from build123d import *

# Parameters (mm, degrees)
SKETCH1_R           = 3.25
BOSS_EXTRUDE1_DEPTH = 6
FILLET1_R           = 0.5
SCALE_1_SCALE       = 2


with BuildPart() as part:
    # Sketch1 → Boss-Extrude1 (new body)
    with BuildSketch(Plane.XY):
        with BuildLine():
            Line((-50.218340611, 5), (149.781659389, 5))
            ThreePointArc((149.781659389, 5), (154.781659389, 0), (149.781659389, -5))
            Line((149.781659389, -5), (-50.218340611, -5))
            ThreePointArc((-50.218340611, -5), (-55.218340611, 0), (-50.218340611, 5))
        make_face()
        with Locations((-50.218340611, 0)):
            Circle(SKETCH1_R, mode=Mode.SUBTRACT)
        with Locations((149.781659389, 0)):
            Circle(SKETCH1_R, mode=Mode.SUBTRACT)
    extrude(amount=BOSS_EXTRUDE1_DEPTH)

    # Fillet1
    fillet1_edges = [part.edges().sort_by_distance(p)[0] for p in [
        (154.781659389, 0, 6),
        (49.781659389, 5, 6),
        (-55.218340611, 0, 6),
        (49.781659389, 5, 0),
        (154.781659389, 0, 0),
        (49.781659389, -5, 0),
        (-55.218340611, 0, 0),
        (49.781659389, -5, 6),
    ]]
    fillet(fillet1_edges, radius=FILLET1_R)


with BuildPart() as part_1:
    # 缩放比例1: scaled about (49.781659389, 0, 3)
    add(part.part.scale(SCALE_1_SCALE).moved(Location((-49.781659389, 0, -3))))


solid = part_1.part
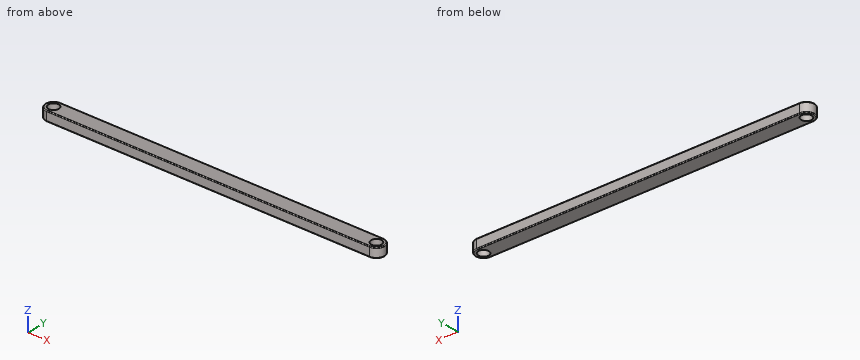
Part model, mm, in its own coordinate system. Round coordinates to 2 decimals unless told otherwise and drop trailing zeros. Write each loop counter-clockwise with the first axis right and the second up, starting at its lowest first coordinate (ties: lowest second). Pieces come first, ordered by that corner, then holes. Notation, with made-up numbers: (56, 33.25) - (82, 33.25) arc R11 ccw to (82, 38.25) - close; hole circle Ø10 at (-26, 35). An arc over 180 degrees is marked (long way). Use CSV: the item, a comma, the result in double quotes.
Item 1: Slice it at B-B, the plane z = 5.75. Write the cut outline in (x, y).
Results list:
outline,"(-150.22, -10) - (249.78, -10) arc R10 ccw to (249.78, 10) - (-150.22, 10) arc R10 ccw to start; hole circle Ø13 at (-150.22, 0); hole circle Ø13 at (249.78, 0)"
Item 2: Flat gauge pins, fed straight in: P1, Ø2, axis at y = -6.5, z = 6.5, coming from the -X side; P2, Ø3, axis at y = 4, z = 4.5, coming from the +X side; P3, Ø1.5, axis at y = 5.5, z = 6.5, coming from the +X side; P4, Ø11.5, axis at x = -150.22, y = 0, coming from the -Z side. Where does each tip first touch, or does it go through?
Results list:
P1,"stops at x = -158.57"
P2,"stops at x = 259.46"
P3,"stops at x = 258.58"
P4,"passes through"
Item 3: Wall check: L1, parallel to X at y = 3.5, z = 7; L2, parallel to X at y = -1.25, z = 2.5; L3, parallel to X at y = -8.75, z = 1. Give the ranges that are in metal, low to high.
Results list:
L1,"x = -159.59 to -155.7, -144.74 to 244.3, 255.26 to 259.15"
L2,"x = -160.14 to -156.6, -143.84 to 243.4, 256.16 to 259.7"
L3,"x = -155.06 to 254.62"
Item 4: Slice it at A-A, the plane y = 0. Write the cut outline in (x, z).
Results list:
outline,"(-160.22, -2) arc R1 ccw to (-159.22, -3) - (-156.72, -3) - (-156.72, 9) - (-159.22, 9) arc R1 ccw to (-160.22, 8) - close; (-143.72, -3) - (243.28, -3) - (243.28, 9) - (-143.72, 9) - close; (256.28, -3) - (258.78, -3) arc R1 ccw to (259.78, -2) - (259.78, 8) arc R1 ccw to (258.78, 9) - (256.28, 9) - close"
